Can you work these out from the drawing? Everything is in mm from the part's minimum corner. Round coordinates to 2 decimals unless told otherwise and drop trailing zeros. Order: outer loops, then holes, each group sorted by start corner. A loop starts at its lowest first (then second) coordinate and runs counter-clockwise, first axis right, second up. Notation, with made-up numbers: M -10.5,82.5 L 13.5,82.5 A13 ccw 13.5,98.5 Z; hole C 77,50 d9. An arc over 180 degrees is marked long. Write item = value, one per line. Start each with the question number.
Item 1: I want a section at B-B, the plane z = 11.5. List the corners of the cut face in (x, y) for me, plus the area to 3 significant figures.
Item 2: I want a section at A-A, the plane z = 41. List the corners of the cut face in (x, y) for me, plus the area to 3 significant figures.
Item 3: I'm going to push flat-ended pins straight in: P1, Ø2, axis at y = 15, z = 41, coming from the -X side; P2, Ø5, axis at x = 5.5, z = 17, coming from the -Y side; P3, Ø8, axis at x = 4.5, z = 5.5, coming from the -Y side. Where does each tip first touch, or does it pass through?
Item 4: Please list where these lines run through material, in increasing order: L1, parallel to X at y = 9, z = 6.25; L2, parallel to X at y = 7.75, z = 5; L3, parallel to Z at x = 12.75, y = 1.
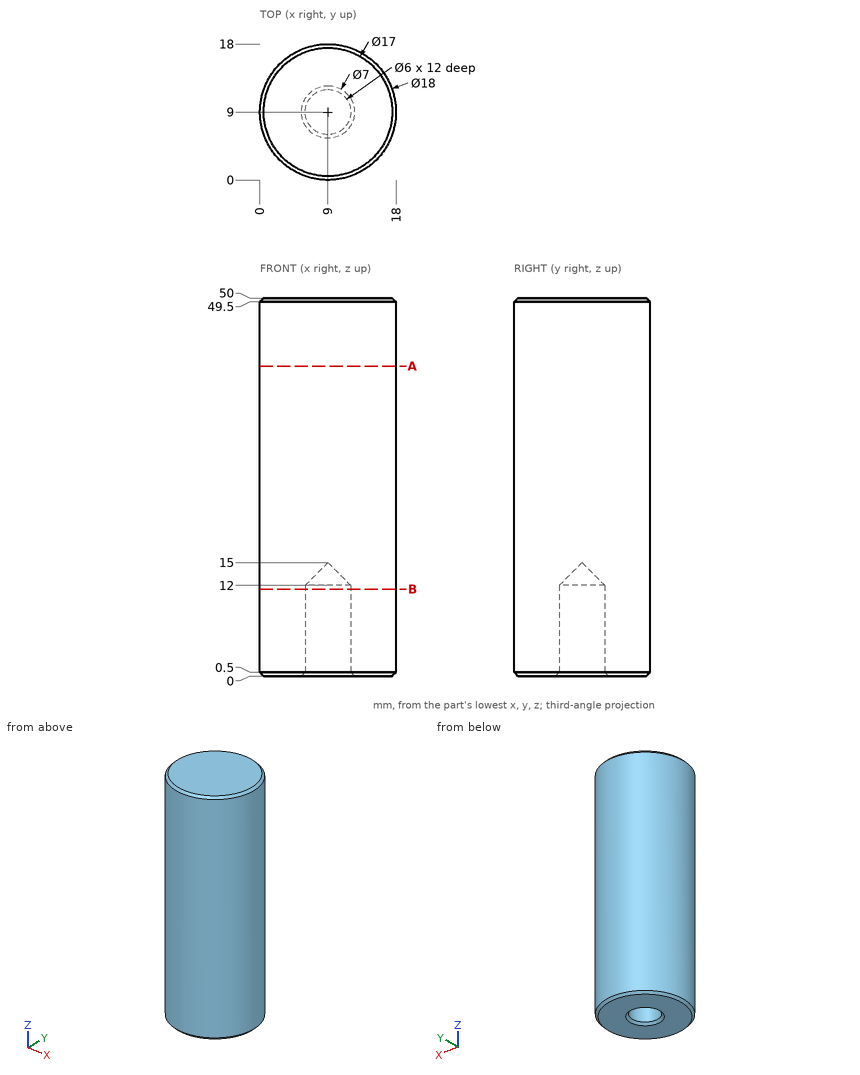
Filled in:
q1.outline = C 9,9 d18; hole C 9,9 d6
q1.area = 226 mm^2
q2.outline = C 9,9 d18
q2.area = 254 mm^2
q3.P1 = 1.52
q3.P2 = 0.06
q3.P3 = 0.01
q4.L1 = 0 to 6, 12 to 18
q4.L2 = 0.09 to 6.27, 11.73 to 17.91
q4.L3 = 0.34 to 49.66
